Could you check a few things on this model? Use its own coordinates, in mm. Face numbers are marked on the shaded views. Round coordinates to 2 decimals unless told otherwise and drop trailing zeros. Loops run counter-clockwise (first coordinate to the right, second up) from the corner with the lowest first, then second, coordinate; pieces in that order, holes last. Notation, with made-up numbers: (-39.75, -7.5) - (-30.75, -7.5) arc R14 ccw to (-30.75, 11.5) - close; hole circle Ø6 at (-8, 61.25). An arc over 180 degrees is marked (long way). Put each result on its own line as item: value. Start each with the question number.
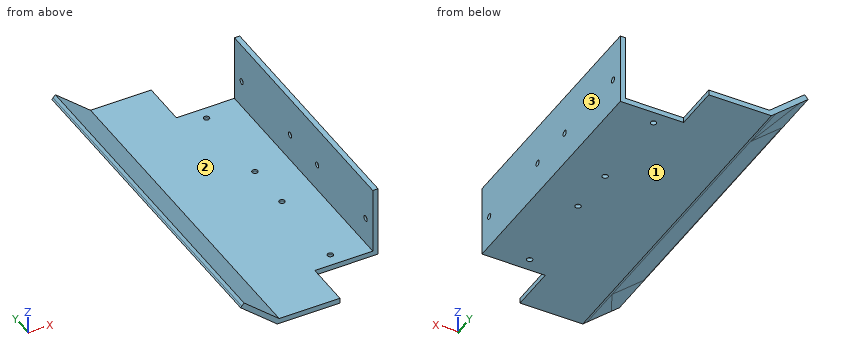
from build123d import *

# Parameters (mm, degrees)
SALIENTE_EXTRUIR1_DEPTH    = 143
CORTAR_EXTRUIR1_REACH      = 91.714
CROQUIS2_R                 = 1.625
CORTAR_EXTRUIR2_REACH      = 38.5
CROQUIS3_R                 = 1.625
CROQUIS4_W                 = 7.355559709
CROQUIS4_H                 = 144.434060974
CORTAR_EXTRUIR3_DEPTH      = 30
SALIENTE_EXTRUIR2_DEPTH    = 1
CROQUIS6_W                 = 1
CROQUIS6_H                 = 143
SALIENTE_EXTRUIR3_DEPTH    = 3.5
SALIENTE_EXTRUIR4_DEPTH    = 26
SALIENTE_EXTRUIR5_DEPTH    = 26
SALIENTE_EXTRUIR6_DEPTH    = 195
CROQUIS10_R                = 1.625
SALIENTE_EXTRUIR7_DEPTH    = 2
CORTAR_EXTRUIR4_DEPTH      = 1
CORTAR_EXTRUIR4_DEPTH_BACK = 196
CROQUIS12_W                = 41
CROQUIS12_H                = 143
CROQUIS12_R                = 1.625
SALIENTE_EXTRUIR8_DEPTH    = 2


with BuildPart() as part:
    # Croquis1 → Saliente-Extruir1 (new body)
    with BuildSketch(Plane(origin=(0, 0, 0), x_dir=(1, 0, 0), z_dir=(0, 1, 0))):
        Polygon((0, 0), (18, 0), (18, 36.5), (-53.969911232, 36.5), (-71.714014286, 21.29146431), (-71.063240069, 20.532193003), (-53.6, 35.5), (17, 35.5), (17, 1), (0, 1), align=None)
    extrude(amount=SALIENTE_EXTRUIR1_DEPTH)

    # Croquis2 → Cortar-Extruir1 (cut, up to next)
    with BuildSketch(Plane(origin=(18, 0, 0), x_dir=(0, 0, -1), z_dir=(1, 0, 0)), mode=Mode.PRIVATE) as cortar_extruir1_sk1:
        with Locations((20, 135.5)):
            Circle(CROQUIS2_R)
    cortar_extruir1_tool1 = extrude(cortar_extruir1_sk1.sketch, amount=-CORTAR_EXTRUIR1_REACH, mode=Mode.PRIVATE) & part.part
    add(cortar_extruir1_tool1.solids().sort_by_distance((18, 135.5, -20))[0], mode=Mode.SUBTRACT)
    # Croquis2 → Cortar-Extruir1 (cut, up to next)
    with BuildSketch(Plane(origin=(18, 0, 0), x_dir=(0, 0, -1), z_dir=(1, 0, 0)), mode=Mode.PRIVATE) as cortar_extruir1_sk2:
        with Locations((20, 7.5)):
            Circle(CROQUIS2_R)
    cortar_extruir1_tool2 = extrude(cortar_extruir1_sk2.sketch, amount=-CORTAR_EXTRUIR1_REACH, mode=Mode.PRIVATE) & part.part
    add(cortar_extruir1_tool2.solids().sort_by_distance((18, 7.5, -20))[0], mode=Mode.SUBTRACT)
    # Croquis2 → Cortar-Extruir1 (cut, up to next)
    with BuildSketch(Plane(origin=(18, 0, 0), x_dir=(0, 0, -1), z_dir=(1, 0, 0)), mode=Mode.PRIVATE) as cortar_extruir1_sk3:
        with Locations((20, 85.5)):
            Circle(CROQUIS2_R)
    cortar_extruir1_tool3 = extrude(cortar_extruir1_sk3.sketch, amount=-CORTAR_EXTRUIR1_REACH, mode=Mode.PRIVATE) & part.part
    add(cortar_extruir1_tool3.solids().sort_by_distance((18, 85.5, -20))[0], mode=Mode.SUBTRACT)
    # Croquis2 → Cortar-Extruir1 (cut, up to next)
    with BuildSketch(Plane(origin=(18, 0, 0), x_dir=(0, 0, -1), z_dir=(1, 0, 0)), mode=Mode.PRIVATE) as cortar_extruir1_sk4:
        with Locations((20, 57.5)):
            Circle(CROQUIS2_R)
    cortar_extruir1_tool4 = extrude(cortar_extruir1_sk4.sketch, amount=-CORTAR_EXTRUIR1_REACH, mode=Mode.PRIVATE) & part.part
    add(cortar_extruir1_tool4.solids().sort_by_distance((18, 57.5, -20))[0], mode=Mode.SUBTRACT)

    # Croquis3 → Cortar-Extruir2 (cut, up to next)
    with BuildSketch(Plane(origin=(0, 0, -36.5), x_dir=(-1, 0, 0), z_dir=(0, 0, -1)), mode=Mode.PRIVATE) as cortar_extruir2_sk1:
        with Locations((3, 7.5)):
            Circle(CROQUIS3_R)
    cortar_extruir2_tool1 = extrude(cortar_extruir2_sk1.sketch, amount=-CORTAR_EXTRUIR2_REACH, mode=Mode.PRIVATE) & part.part
    add(cortar_extruir2_tool1.solids().sort_by_distance((-3, 7.5, -36.5))[0], mode=Mode.SUBTRACT)
    # Croquis3 → Cortar-Extruir2 (cut, up to next)
    with BuildSketch(Plane(origin=(0, 0, -36.5), x_dir=(-1, 0, 0), z_dir=(0, 0, -1)), mode=Mode.PRIVATE) as cortar_extruir2_sk2:
        with Locations((3, 135.5)):
            Circle(CROQUIS3_R)
    cortar_extruir2_tool2 = extrude(cortar_extruir2_sk2.sketch, amount=-CORTAR_EXTRUIR2_REACH, mode=Mode.PRIVATE) & part.part
    add(cortar_extruir2_tool2.solids().sort_by_distance((-3, 135.5, -36.5))[0], mode=Mode.SUBTRACT)
    # Croquis3 → Cortar-Extruir2 (cut, up to next)
    with BuildSketch(Plane(origin=(0, 0, -36.5), x_dir=(-1, 0, 0), z_dir=(0, 0, -1)), mode=Mode.PRIVATE) as cortar_extruir2_sk3:
        with Locations((3, 57.5)):
            Circle(CROQUIS3_R)
    cortar_extruir2_tool3 = extrude(cortar_extruir2_sk3.sketch, amount=-CORTAR_EXTRUIR2_REACH, mode=Mode.PRIVATE) & part.part
    add(cortar_extruir2_tool3.solids().sort_by_distance((-3, 57.5, -36.5))[0], mode=Mode.SUBTRACT)
    # Croquis3 → Cortar-Extruir2 (cut, up to next)
    with BuildSketch(Plane(origin=(0, 0, -36.5), x_dir=(-1, 0, 0), z_dir=(0, 0, -1)), mode=Mode.PRIVATE) as cortar_extruir2_sk4:
        with Locations((3, 85.5)):
            Circle(CROQUIS3_R)
    cortar_extruir2_tool4 = extrude(cortar_extruir2_sk4.sketch, amount=-CORTAR_EXTRUIR2_REACH, mode=Mode.PRIVATE) & part.part
    add(cortar_extruir2_tool4.solids().sort_by_distance((-3, 85.5, -36.5))[0], mode=Mode.SUBTRACT)

    # Croquis4 → Cortar-Extruir3 (cut)
    with BuildSketch(Plane(origin=(18, 0, 0), x_dir=(0, 0, -1), z_dir=(1, 0, 0))):
        with Locations((-2.677779855, 72.217030487)):
            Rectangle(CROQUIS4_W, CROQUIS4_H)
    extrude(amount=-CORTAR_EXTRUIR3_DEPTH, mode=Mode.SUBTRACT)

    # Croquis5 → Saliente-Extruir2 (add)
    with BuildSketch(Plane(origin=(-40.891807576, 0, -47.709290524), x_dir=(-0.759271307, 0, 0.650774217), z_dir=(-0.650774217, 0, -0.759271307))):
        Polygon((17.224546128, 0), (35.59445736, -26), (40.59445736, -26), (40.59445736, 0), (17.59445736, 0), align=None)
        Polygon((40.59445736, 143), (17.59445736, 143), (17.224546128, 143), (35.59445736, 169), (40.59445736, 169), align=None)
    extrude(amount=-SALIENTE_EXTRUIR2_DEPTH)

    # Croquis6 → Saliente-Extruir3 (add)
    with BuildSketch(Plane.XY.offset(-1)):
        with Locations((17.5, 71.5)):
            Rectangle(CROQUIS6_W, CROQUIS6_H)
    extrude(amount=SALIENTE_EXTRUIR3_DEPTH)

    # Croquis7 → Saliente-Extruir4 (add)
    with BuildSketch(Plane.XZ.offset(26)):
        Polygon((-67.266883532, -23.786064089), (-67.917657749, -24.545335397), (-53.972777222, -36.497543549), (-53.969911232, -36.5), (-16, -36.5), (-16, -35.5), (-53.6, -35.5), align=None)
    extrude(amount=-SALIENTE_EXTRUIR4_DEPTH)

    # Croquis8 → Saliente-Extruir5 (add)
    with BuildSketch(Plane(origin=(0, 169, 0), x_dir=(1, 0, 0), z_dir=(0, 1, 0))):
        Polygon((-67.917657749, 24.545335397), (-53.969911232, 36.5), (-16, 36.5), (-16, 35.5), (-53.595402654, 35.5), (-67.264936524, 23.783792475), align=None)
    extrude(amount=-SALIENTE_EXTRUIR5_DEPTH)

    # Croquis9 → Saliente-Extruir6 (add)
    with BuildSketch(Plane(origin=(0, 169, 0), x_dir=(1, 0, 0), z_dir=(0, 1, 0))):
        Polygon((-71.714014286, 21.29146431), (-71.063240069, 20.532193003), (-53.595402654, 35.5), (-50.526737497, 35.5), (-70.520962942, 18.362876171), (-71.822511376, 19.881418786), (-72.473285593, 20.640690093), align=None)
    extrude(amount=-SALIENTE_EXTRUIR6_DEPTH)

    # Croquis10 → Saliente-Extruir7 (add)
    with BuildSketch(Plane(origin=(0, 0, -36.5), x_dir=(-1, 0, 0), z_dir=(0, 0, -1))):
        Polygon((-18, 0), (16, 0), (16, -26), (53.969911232, -26), (53.969911232, 169), (16, 169), (16, 143), (-18, 143), align=None)
        with Locations((3, 7.5)):
            Circle(CROQUIS10_R, mode=Mode.SUBTRACT)
        with Locations((3, 57.5)):
            Circle(CROQUIS10_R, mode=Mode.SUBTRACT)
        with Locations((3, 85.5)):
            Circle(CROQUIS10_R, mode=Mode.SUBTRACT)
        with Locations((3, 135.5)):
            Circle(CROQUIS10_R, mode=Mode.SUBTRACT)
    extrude(amount=SALIENTE_EXTRUIR7_DEPTH)

    # Croquis11 → Cortar-Extruir4 (cut, two sides)
    with BuildSketch(Plane.XZ.offset(26)) as cortar_extruir4_sk:
        Polygon((-53.969911232, -36.5), (-51.636471194, -38.5), (-54.241943892, -38.819087413), align=None)
    extrude(amount=CORTAR_EXTRUIR4_DEPTH, mode=Mode.SUBTRACT)
    extrude(cortar_extruir4_sk.sketch, amount=-CORTAR_EXTRUIR4_DEPTH_BACK, mode=Mode.SUBTRACT)

    # Croquis12 → Saliente-Extruir8 (add)
    with BuildSketch(Plane(origin=(18, 0, 0), x_dir=(0, 0, -1), z_dir=(1, 0, 0))):
        with Locations((18, 71.5)):
            Rectangle(CROQUIS12_W, CROQUIS12_H)
        with Locations((20, 7.5)):
            Circle(CROQUIS12_R, mode=Mode.SUBTRACT)
        with Locations((20, 57.5)):
            Circle(CROQUIS12_R, mode=Mode.SUBTRACT)
        with Locations((20, 85.5)):
            Circle(CROQUIS12_R, mode=Mode.SUBTRACT)
        with Locations((20, 135.5)):
            Circle(CROQUIS12_R, mode=Mode.SUBTRACT)
    extrude(amount=SALIENTE_EXTRUIR8_DEPTH)


solid = part.part
Item 1: Will these pins go through, and if not, where does the flat tip stop? P1, Ø2.5, axis at y = 135.5, z = -20, coming from the +X side; P2, Ø19, axis at y = 48.5, z = -21.5, coming from the -X side; P3, Ø20.5, axis at x = -3.5, y = 63, coming from the +Z side.
Item 2: I need wall thicknesses on line 1 (Y direction, x = -3, z = -37) (3 decimals); line 2 (Z direction, x = -18, y = 53); line 3 (X direction, y = 49, z = -5). Which ranges of each line are inside material? Lowest first, please. Write a range as from..to.
Item 3: Suppose I cut it at C-C, the plane z = -4.5. List the corners of the cut face in (x, y) for me, then the cut area to 3 significant figures.
Item 4: Suppose I cut it at D-D, the plane x = -35. List the corners of the cut face in (y, z) for me, then the cut area to 3 significant figures.
Item 5: Thinking about a two-plate mould opening in X: for the marked faces 1, 2 and 3, which applies, released by +X, released by -X, zero draft, split by the parting line, or undercut?
Numbers:
1. P1: x = -67.15
1. P2: x = -72.47
1. P3: z = -35.5
2. line 1: 0..5.875, 9.125..55.875, 59.125..83.875, 87.125..133.875, 137.125..143
2. line 2: -38.5..-35.5
2. line 3: 17..20
3. outline: (17, 0) - (20, 0) - (20, 143) - (17, 143) - close
3. area: 429 mm^2
4. outline: (-26, -38.5) - (169, -38.5) - (169, -35.5) - (-26, -35.5) - close
4. area: 585 mm^2
5. face 1: zero draft
5. face 2: undercut
5. face 3: released by +X
